Autodesk Inventor part; units mm, degrees
ref_plane "YZ Plane" through (0, 0, 0) normal (1, 0, 0) x (0, 1, 0)
ref_plane "XZ Plane" through (0, 0, 0) normal (0, 1, 0) x (-1, 0, 0)
ref_plane "XY Plane" through (0, 0, 0) normal (0, 0, 1) x (1, 0, 0)
sketch "Sketch1" plane through (0, 0, 0) normal (0, 0, 1) x (1, 0, 0)
  line L0 (0, 0) -> (400, 0)
  line L1 (400, 0) -> (400, 600)
  line L2 (400, 600) -> (0, 600)
  line L3 (0, 600) -> (0, 0)
  dimension "d0" = 400
  dimension "d1" = 600
extrude "Extrusion1" add sketch "Sketch1" along normal blind 3
sketch "Sketch2" plane through (0, 0, 3) normal (0, 0, 1) x (1, 0, 0)
  line L0 (400, 600) -> (0, 600)
  line L1 (400, 0) -> (400, 600)
  line L2 (0, 600) -> (400, 600)
  line L3 (400, 600) -> (400, 0)
  line L4 (400, 0) -> (0, 0)
  line L5 (0, 0) -> (0, 600)
  line L6 (3, 597) -> (397, 597)
  line L7 (397, 597) -> (397, 3)
  line L8 (397, 3) -> (3, 3)
  line L9 (3, 3) -> (3, 597)
  dimension "d4" = 3
extrude "Extrusion2" add sketch "Sketch2" along normal blind 250
sketch "Sketch3" plane through (3, 597, 3) normal (0, -1, 0) x (1, 0, 0)
  line L0 (54, 110) -> (114, 110)
  line L1 (114, 110) -> (114, 70)
  line L2 (114, 70) -> (54, 70)
  line L3 (54, 70) -> (54, 110)
  line L4 (0, 250) -> (394, 250)
  line L5 (394, 0) -> (0, 0)
  point P0 (-3, -3)
  dimension "d7" = 40
  dimension "d8" = 60
  dimension "d9" = 54
  dimension "d11" = 70
extrude "Extrusion3" add sketch "Sketch3" along normal blind 40
sketch "Sketch4" plane through (3, 557, 3) normal (0, -1, 0) x (1, 0, 0)
  circle A0 centre (104, 90) radius 5
  line L0 (114, 70) -> (114, 110)
  line L1 (114, 110) -> (54, 110)
  point P0 (-3, -3)
  dimension "d14" = 10
  dimension "d15" = 10
  dimension "d16" = 20
extrude "Extrusion4" add sketch "Sketch4" along normal blind 30
sketch "Sketch5" plane through (0, 0, 253) normal (0, 0, 1) x (1, 0, 0)
  line L0 (3, 3) -> (3, 597)
  line L1 (3, 557) -> (23, 557)
  line L2 (23, 557) -> (23, 527)
  line L3 (23, 527) -> (3, 527)
  line L4 (3, 527) -> (3, 557)
  line L5 (23, 544.5) -> (18, 544.5)
  line L6 (18, 544.5) -> (18, 539.5)
  line L7 (18, 539.5) -> (23, 539.5)
  line L8 (23, 539.5) -> (23, 544.5)
  line L9 (23, 542) -> (-4.5465, 542) construction
  line L10 (18, 552) -> (13, 552)
  line L11 (13, 552) -> (13, 532)
  line L12 (13, 532) -> (18, 532)
  line L13 (18, 532) -> (18, 552)
  line L14 (3, 597) -> (397, 597) construction
  point P0 (0, 0)
  point P1 (18, 542)
  point P2 (18, 544.5)
  point P3 (3, 527)
  point P4 (23, 539.5)
  point P5 (18, 539.5)
  dimension "d19" = 20
  dimension "d20" = 30
  dimension "d21" = 5
  dimension "d22" = 5
  dimension "d24" = 2.5
  dimension "d25" = 5
  dimension "d26" = 20
  dimension "d28" = 10
  dimension "d29" = 40
extrude "Extrusion5" add sketch "Sketch5" against normal blind 250 contours L0 L1 L2 L5 L13 L10 L11 L12 L7 L3
sketch "Sketch6" plane through (0, 0, 3) normal (0, 0, 1) x (1, 0, 0)
  line L0 (148, 497) -> (193, 497)
  line L1 (193, 497) -> (193, 377)
  line L2 (193, 377) -> (148, 377)
  line L3 (148, 377) -> (148, 497)
  line L4 (3, 3) -> (3, 527)
  line L5 (3, 597) -> (397, 597)
  point P0 (0, 0)
  dimension "d32" = 45
  dimension "d33" = 120
  dimension "d34" = 145
  dimension "d35" = 100
extrude "Extrusion6" add sketch "Sketch6" along normal blind 5
sketch "Sketch7" plane through (0, 0, 8) normal (0, 0, 1) x (1, 0, 0)
  line L0 (148, 377) -> (193, 377)
  line L1 (148, 497) -> (193, 497)
  line L2 (193, 497) -> (193, 377)
  line L3 (193, 377) -> (148, 377)
  line L4 (148, 377) -> (148, 497)
  line L5 (191, 495) -> (150, 495)
  line L6 (150, 495) -> (150, 379)
  line L7 (150, 379) -> (191, 379)
  line L8 (191, 379) -> (191, 495)
  point P0 (0, 0)
  point P1 (148, 377)
  dimension "d40" = 2
extrude "Extrusion7" add sketch "Sketch7" along normal blind 5 contours L8 L7 L6 L5
sketch "Sketch8" plane through (0, 0, 253) normal (0, 0, 1) x (1, 0, 0)
  line L0 (3, 527) -> (3, 3)
  line L1 (53, 26) -> (63, 26)
  line L2 (63, 26) -> (63, 6)
  line L3 (63, 6) -> (53, 6)
  line L4 (53, 6) -> (53, 26)
  line L5 (397, 3) -> (3, 3)
  line L6 (153, 26) -> (163, 26)
  line L7 (163, 26) -> (163, 6)
  line L8 (163, 6) -> (153, 6)
  line L9 (153, 6) -> (153, 26)
  line L10 (58, 16) -> (63, 16)
  line L11 (63, 16) -> (63, 11)
  line L12 (63, 11) -> (58, 11)
  line L13 (58, 11) -> (58, 16)
  line L14 (153, 16) -> (158, 16)
  line L15 (158, 16) -> (158, 11)
  line L16 (158, 11) -> (153, 11)
  line L17 (153, 11) -> (153, 16)
  point P0 (0, 0)
  point P1 (53, 28)
  dimension "d54" = 10
  dimension "d55" = 20
  dimension "d57" = 50
  dimension "d60" = 3
  dimension "d61" = 10
  dimension "d62" = 20
  dimension "d65" = 3
  dimension "d74" = 5
  dimension "d75" = 5
  dimension "d76" = 90
  dimension "d77" = 5
  dimension "d79" = 5
  dimension "d80" = 5
  dimension "d81" = 5
extrude "Extrusion8" add sketch "Sketch8" against normal blind 210 contours L1 L2 L10 L13 L12 L3 L4 | L6 L7 L8 L9 L16 L15 L14
sketch "Sketch9" plane through (53, 6, 253) normal (0, -1, 0) x (1, 0, 0)
  line L0 (0, 0) -> (0, -210)
  line L1 (10, 0) -> (10, -210)
  line L2 (0, 0) -> (10, 0)
  line L3 (10, 0) -> (10, -10)
  line L4 (10, -10) -> (0, -10)
  line L5 (0, -10) -> (0, 0)
  line L6 (100, 0) -> (110, 0)
  line L7 (110, 0) -> (110, -210)
  line L8 (100, 0) -> (110, 0)
  line L9 (110, 0) -> (110, -10)
  line L10 (110, -10) -> (100, -10)
  line L11 (100, -10) -> (100, 0)
  line L12 (10, -210) -> (0, -210)
  line L13 (0, -210) -> (10, -210)
  line L14 (10, -210) -> (10, -200)
  line L15 (10, -200) -> (0, -200)
  line L16 (0, -200) -> (0, -210)
  line L17 (110, -210) -> (100, -210)
  line L18 (100, -210) -> (110, -210)
  line L19 (110, -210) -> (110, -200)
  line L20 (110, -200) -> (100, -200)
  line L21 (100, -200) -> (100, -210)
  point P0 (-53, -253)
  point P1 (10, -200)
  point P2 (0, -200)
  dimension "d67" = 10
  dimension "d68" = 10
  dimension "d69" = 10
  dimension "d70" = 10
  dimension "d73" = 10
extrude "Extrusion9" add sketch "Sketch9" along normal blind 3 contours L2 L1 L4 L0 | L15 L1 L12 L0 | L7 L17 L21 L20 | L6 L7 L10 L11
sketch "Sketch10" plane through (3, 3, 3) normal (0, 1, 0) x (1, 0, 0)
  line L0 (90, -90) -> (120, -90)
  line L1 (120, -90) -> (120, -190)
  line L2 (120, -190) -> (90, -190)
  line L3 (90, -190) -> (90, -90)
  line L4 (50, -50) -> (60, -50)
  line L5 (60, -240) -> (50, -240)
  line L6 (60, -250) -> (60, -40)
  point P0 (-3, 3)
  dimension "d84" = 30
  dimension "d85" = 100
  dimension "d87" = 50
  dimension "d88" = 30
extrude "Extrusion10" cut sketch "Sketch10" against normal blind 5
sketch "Sketch11" plane through (3, 3, 3) normal (0, 1, 0) x (1, 0, 0)
  line L0 (130, -130) -> (135, -130)
  line L1 (135, -130) -> (135, -150)
  line L2 (135, -150) -> (130, -150)
  line L3 (130, -150) -> (130, -130)
  line L4 (120, -90) -> (120, -190)
  line L5 (120, -190) -> (90, -190)
  point P0 (-3, 3)
  dimension "d91" = 5
  dimension "d92" = 20
  dimension "d93" = 10
  dimension "d94" = 40
extrude "Extrusion11" add sketch "Sketch11" along normal blind 3
sketch "Sketch12" plane through (0, 0, 3) normal (0, 0, 1) x (1, 0, 0)
  line L0 (120.5173, 297) -> (317, 187.3663)
  line L1 (317, 187.3663) -> (314.5637, 183)
  line L2 (314.5637, 183) -> (118.081, 292.6337)
  line L3 (120.5173, 297) -> (118.081, 292.6337)
  line L4 (397, 597) -> (397, 3)
  line L5 (397, 3) -> (3, 3)
  line L6 (3, 597) -> (397, 597)
  point P0 (0, 0)
  point P1 (163, 3)
  dimension "d97" = 5
  dimension "d99" = 80
  dimension "d100" = 180
  dimension "d101" = 225
  dimension "d104" = 300
extrude "Extrusion12" add sketch "Sketch12" along normal blind 150
sketch "Sketch13" plane through (3, 597, 3) normal (0, -1, 0) x (1, 0, 0)
  line L0 (174, 110) -> (214, 110)
  line L1 (214, 110) -> (214, 70)
  line L2 (214, 70) -> (174, 70)
  line L3 (174, 70) -> (174, 110)
  circle A0 centre (104, 90) radius 5
  point P0 (-3, -3)
  dimension "d105" = 40
  dimension "d106" = 70
extrude "Extrusion13" add sketch "Sketch13" along normal blind 40 contours L0 L1 L2 L3
sketch "Sketch15" plane through (3, 557, 3) normal (0, -1, 0) x (1, 0, 0)
  circle A0 centre (194, 90) radius 5
  circle A1 centre (194, 90) radius 2.5
  line L0 (174, 110) -> (174, 70)
  line L1 (214, 110) -> (174, 110)
  point P0 (-3, -3)
  dimension "d114" = 10
  dimension "d115" = 5
  dimension "d116" = 20
  dimension "d117" = 20
extrude "Extrusion15" add sketch "Sketch15" along normal blind 5
sketch "Sketch16" plane through (0, 0, 3) normal (0, 0, 1) x (1, 0, 0)
  circle A0 centre (183, 68) radius 5
  circle A1 centre (367, 68) radius 5
  line L0 (397, 597) -> (397, 3)
  line L1 (163, 3) -> (163, 26)
  line L2 (397, 3) -> (163, 3)
  circle A2 centre (273, 68) radius 5
  point P0 (0, 0)
  dimension "d120" = 10
  dimension "d121" = 10
  dimension "d122" = 30
  dimension "d123" = 20
  dimension "d124" = 65
  dimension "d125" = 65
  dimension "d128" = 10
  dimension "d129" = 90
extrude "Extrusion16" add sketch "Sketch16" along normal blind 250
sketch "Sketch17" plane through (120.5173, 297, 153) normal (0.4873, 0.8733, 0) x (0.8733, -0.4873, 0)
  line L0 (225, 150) -> (225, 0)
  line L1 (225, 59.1442) -> (16.5288, 150)
  line L2 (-214.6928, 150) -> (40.632, 150)
  line L3 (11.5288, 150) -> (225, 54.1442)
  line L4 (225, 54.1442) -> (225, 59.1442)
  line L5 (11.5288, 150) -> (16.5288, 150)
  point P0 (39.474, 153)
  dimension "d132" = 5
  dimension "d133" = 5
extrude "Extrusion17" add sketch "Sketch17" along normal blind 20
properties part number "caja"
Source: CAD feature listing. Evaluate the final solid. Frame: model axes, mm. A direction names the side the tool comes from. Coordinates: 2 decimals unless noted, no trailing zeros. Write each loop counter-clockwise with the first axis right and the second up, starting at its lowest first coordinate (ties: lowest second). Pieces come first, ordered by that corner, then holes. Notation, with made-up numbers: (43, -0.75) -> (76, -0.75) arc R26 ccw to (76, 37.25) -> close; hole circle Ø2 at (16, -30). An arc over 180 degrees is marked (long way). Return JSON: item names as keys, results as strings. Group by question number.
1) Section query A-A, the plane z = 31. State how many separate pieces and enclosed holes the cut face has, plus the area to 3 significant figures.
2) Ray query, line 1 along Y through (x, z) = (21.5, 117); line 2 along Y through (x, z) = (360, 30.5); line 3 along X through (y, z) = (92, 214.5). Return the intervals inside material, ascending.
3) Set-up query: faces 1 (the face through (23, 551, 130)), 2 (the face through (232.054, 246.054, 49.064)). Return all of +Z, -Z, +X, -X, +Y, -Y with unobstructed straight access to the full face (end or side cutting, diameter ignored); none if empty.
4) Section query B-B, the plane y = 360.5. Return loops of the section in (x, z), plus the area to 3 significant figures.
5) Mould query, pull axis X, two halves, no side actions, for faces 3 (the face through (217.7, 237.05, 76.95)), 4 (the face through (0, 304, 125)), 5 (the face through (13, 542, 130)), 6 (the face through (197, 0, 125)). Classes: +X half, -X half, draft (parallel to the pull), parting line (faces both ways), or undercut.
6) Contact query for a flat-ended pin moving along its axis: P1, Ø12, axis at x = 92, y = 468.5, coming from the +Z side. Output: stop coordinate, or through.
From the geometry:
{
 "1": {"separate pieces": "5", "enclosed holes": "1", "area": "7,940 mm²"},
 "2": {"line 1": "0 to 3, 527 to 539.5, 544.5 to 557, 597 to 600", "line 2": "0 to 3, 597 to 600", "line 3": "0 to 3, 397 to 400"},
 "3": {"face 1": "+Z", "face 2": "none"},
 "4": {"outline": "(0, 0) -> (400, 0) -> (400, 253) -> (397, 253) -> (397, 3) -> (3, 3) -> (3, 253) -> (0, 253) -> close", "area": "2,700 mm²"},
 "5": {"face 3": "undercut", "face 4": "-X half", "face 5": "undercut", "face 6": "draft"},
 "6": {"P1": "z = 3"}
}
